```python
from build123d import *

# Parameters (mm, degrees)
SKETCH1_W           = 40
SKETCH1_H           = 40
BOSS_EXTRUDE1_DEPTH = 40
SKETCH2_W           = 20
SKETCH2_H           = 20
CUT_EXTRUDE1_DEPTH  = 40
CUT_EXTRUDE2_DEPTH  = 20
CUT_EXTRUDE4_DEPTH  = 20
CUT_EXTRUDE5_DEPTH  = 20


with BuildPart() as part:
    # Sketch1 → Boss-Extrude1 (new body)
    with BuildSketch(Plane.XY):
        with Locations((20, 20)):
            Rectangle(SKETCH1_W, SKETCH1_H)
    extrude(amount=BOSS_EXTRUDE1_DEPTH)

    # Sketch2 → Cut-Extrude1 (cut)
    with BuildSketch(Plane.XY.offset(40)):
        with Locations((30, 30)):
            Rectangle(SKETCH2_W, SKETCH2_H)
    extrude(amount=-CUT_EXTRUDE1_DEPTH, mode=Mode.SUBTRACT)

    # Sketch3 → Cut-Extrude2 (cut)
    with BuildSketch(Plane(origin=(40, 0, 0), x_dir=(0, 0, -1), z_dir=(1, 0, 0))):
        Polygon((-40, 0), (-20, 20), (-40, 20), align=None)
    extrude(amount=-CUT_EXTRUDE2_DEPTH, mode=Mode.SUBTRACT)

    # Sketch5 → Cut-Extrude4 (cut)
    with BuildSketch(Plane(origin=(0, 0, 0), x_dir=(-1, 0, 0), z_dir=(0, 0, -1))):
        Polygon((-20, 40), (0, 20), (0, 40), align=None)
    extrude(amount=-CUT_EXTRUDE4_DEPTH, mode=Mode.SUBTRACT)

    # Sketch6 → Cut-Extrude5 (cut)
    with BuildSketch(Plane.ZY):
        Polygon((20, 40), (40, 0), (40, 40), align=None)
    extrude(amount=-CUT_EXTRUDE5_DEPTH, mode=Mode.SUBTRACT)


solid = part.part
```
Here's how the part is built. I have some questions about the finished solid (model axes, mm). A direction names the side the tool comes from. Round coordinates to 2 decimals unless told otherwise and drop trailing zeros. Order: outer loops, then holes, each group sorted by start corner. A loop starts at its lowest first (then second) coordinate and runs counter-clockwise, first axis right, second up. Notation, with made-up numbers: M 32.25,-27.75 L 40.25,-27.75 A19 cw 40.25,5.25 Z; hole C 87.25,24 d11. An arc over 180 degrees is marked long. Answer in a Markdown table with one row per item.
Item 1: If I drill on L1, parallel to X at y = 25, z = 25; L2, parallel to Y at x = 26, z = 37, over which ranges is the centre line in solid material (lowest first)? Write a range as from..to.
A:
| item | result |
|---|---|
| L1 | x = 0..20 |
| L2 | y = 0..3 |
Item 2: Imagine slicing it at B-B, the plane x = 18.5. Write out the boundary of the cut face in (y, z), and give its area (3 significant figures).
A:
| item | result |
|---|---|
| outline | M 0,0 L 38.5,0 L 38.5,20 L 40,20 L 0,40 Z |
| area | 1,170 mm2 |
Item 3: Imagine slicing it at A-A, the plane z = 32.5. Write out the boundary of the cut face in (x, y).
A:
| item | result |
|---|---|
| outline | M 0,0 L 40,0 L 40,7.5 L 20,7.5 L 20,15 L 0,15 Z |
Item 4: Imagine slicing it at C-C, the plane y = 33.5. Write out the boundary of the cut face in (x, z).
A:
| item | result |
|---|---|
| outline | M 0,20 L 13.5,20 L 13.5,0 L 20,0 L 20,23.25 L 0,23.25 Z |
Item 5: Imagine slicing it at D-D, the plane x = 14. Write out the boundary of the cut face in (y, z).
A:
| item | result |
|---|---|
| outline | M 0,0 L 34,0 L 34,20 L 40,20 L 0,40 Z |
Item 6: For faces 4 (the face through (10, 30, 10)), 5 (the face through (0, 11, 20)), 6 (the face through (20, 27, 16)), which set-ups out of +Z, -Z, +X, -X, +Y, -Y let a thin tool reach every point of the face, with its end or its side?
A:
| item | result |
|---|---|
| face 4 | -Z, -X, +Y |
| face 5 | +Z, -Z, -X, +Y, -Y |
| face 6 | +Z, +X, +Y |
Item 7: Thinking about a two-plate mould opening in Z: for faces 1 (the face through (30, 20, 10)), 2 (the face through (10, 20, 30)), 3 (the face through (6, 35, 20)), which applies, +Z half, -Z half, draft (parallel to the pull), parting line (faces both ways), or undercut?
A:
| item | result |
|---|---|
| face 1 | draft |
| face 2 | +Z half |
| face 3 | -Z half |
Item 8: I'm going to push flat-ended pins straight in: pin 1 (4 mm diameter, centred on y = 29.5, z = 22.5, fed in from +X); pin 2 (3 mm diameter, centred on x = 10, z = 19, fed in from -Y); pin 3 (10 mm diameter, centred on x = 33.5, z = 34, fed in from +Y); pin 4 (5 mm diameter, centred on x = 25.5, z = 17, fed in from +Y). Where does each tip first touch, or does it pass through?
A:
| item | result |
|---|---|
| pin 1 | stops at x = 20 |
| pin 2 | stops at y = 0 |
| pin 3 | stops at y = 11 |
| pin 4 | stops at y = 20 |
